```python
from build123d import *

# Parameters (mm, degrees)
F1_DEPTH = 25
F2_SIZE2 = 10
F2_SIZE  = 20
F4_DEPTH = 50
F5_T     = -2.5
F6_R     = 1


with BuildPart() as f1:
    # F0 (on Front) → F1 (new body)
    with BuildSketch(Plane.XZ):
        Polygon((63.5576491768, 36.6950258613), (-63.5576491768, 36.6950258613), (0, -73.3900517225), align=None)
    extrude(amount=-F1_DEPTH)

    # F2
    f2_edges = [f1.edges().sort_by_distance(p)[0] for p in [
        (-31.778825, 25, -18.347513),
        (0, 25, 36.695026),
        (31.778825, 25, -18.347513),
    ]]
    f2_side = f1.faces().sort_by_distance((0, 25, 0))[0]
    chamfer(f2_edges, length=F2_SIZE, length2=F2_SIZE2, reference=f2_side)

    # F3 (on face) → F4 (join, symmetric)
    with BuildSketch(Plane(origin=(0, 25, 0), x_dir=(-1, 0, 0), z_dir=(0, 1, 0))):
        Polygon((-10.3546479691, -5.9782587923), (10.3546479691, -5.9782587923), (0, 11.9565175846), align=None)
    extrude(amount=F4_DEPTH, both=True)

    # F5
    f5_openings = [f1.faces().sort_by_distance(p)[0] for p in [
        (0, -25, 0),
    ]]
    offset(amount=F5_T, openings=f5_openings, kind=Kind.INTERSECTION)

    # F6
    f6_edges = [f1.edges().sort_by_distance(p)[0] for p in [
        (0, -25, -5.978259),
        (0, -25, -3.478259),
        (3.01226, -25, 1.739129),
        (5.177324, -25, 2.989129),
        (-5.177324, -25, 2.989129),
        (-3.01226, -25, 1.739129),
    ]]
    fillet(f6_edges, radius=F6_R)


solid = f1.part
```
Source: CAD feature listing. Evaluate the final solid. Frame: model axes, mm. A direction names the side the tool comes from. Coordinates: 2 decimals unless noted, no trailing zeros. Write each loop counter-clockwise with the first axis right and the second up, starting at its lowest first coordinate (ties: lowest second). Pieces come first, ordered by that corner, then holes. Notation, with made-up numbers: (8, -15.5) - (34, -15.5) arc R9 cw to (34, -0.5) - close; hole circle Ø5 at (-6, 60). An arc over 180 degrees is marked (long way). Answer as a JSON object with one key per item and string values.
Q1. Section query C-C, the plane y = -10.5. Output: boundary loops of the cut face in (x, z).
Ans:
{"outline": "(-10.35, -5.98) - (10.35, -5.98) - (0, 11.96) - close; hole (-6.02, -3.48) - (6.02, -3.48) - (0, 6.96) - close"}
Q2. Section query A-A, the plane x = 19. Output: boundary loops of the cut face in (y, z).
Ans:
{"outline": "(0, -40.48) - (15, -40.48) - (25, -0.48) - (25, 16.7) - (15, 36.7) - (0, 36.7) - close; hole (2.5, -35.48) - (13.45, -35.48) - (22.5, 0.7) - (22.5, 16.1) - (13.45, 34.2) - (2.5, 34.2) - close"}
Q3. Section query D-D, the plane z = -59.5. Output: boundary loops of the cut face in (x, y).
Ans:
{"outline": "(-8.02, 0) - (8.02, 0) - (8.02, 15) - (0, 18.47) - (-8.02, 15) - close; hole (-5.13, 2.5) - (5.13, 2.5) - (5.13, 13.45) - (0, 15.68) - (-5.13, 13.45) - close"}
Q4. Set-up query: faces 4 (the flat face through (2.97, -10.56, 1.81)), 5 (the flat face through (-1, 2.5, -5)), 6 (the flat face through (0.89, 18.819, 29.057)), 7 (the flat face through (0, 50, -5.978)), 8 (the flat face through (0, -12, -5.978)). Return all of +Z, -Z, +X, -X, +Y, -Y with unobstructed straight access to the full face (end or side cutting, diameter ignored); none if empty.
Ans:
{"face 4": "-Y", "face 5": "none", "face 6": "+Z, +X, -X, +Y", "face 7": "-Z, +X, -X, +Y", "face 8": "-Z, +X, -X, -Y"}
Q5. Draft query along Z for faces 1 (the flat face through (23.22, 16.91, -14.36)), 2 (the flat face through (-25.61, 18.82, -13.76)), 3 (the flat face through (-7, 25, 3)). Return one class per face: released by +Z, released by -Z, zero draft, split by the parting line, or undercut.
Ans:
{"face 1": "undercut", "face 2": "released by -Z", "face 3": "zero draft"}
Q6. Material intervals for line 1 (Y direction, x = 8, z = 6); line 2 (Y direction, x = -19.5, z = -13.5); line 3 (Y direction, x = -35, z = -8.5), sorted ascending. Write a range as [from, to].
Ans:
{"line 1": "y = [0, 2.5], [22.5, 25]", "line 2": "y = [0, 2.5], [18.73, 21.53]", "line 3": "y = [0, 16.07]"}
Q7. Section query B-B, the plane z = -16. Output: boundary loops of the cut face in (x, y).
Ans:
{"outline": "(-33.13, 0) - (33.13, 0) - (33.13, 15) - (10.04, 25) - (-10.04, 25) - (-33.13, 15) - close; hole (-30.25, 2.5) - (30.25, 2.5) - (30.25, 13.45) - (9.36, 22.5) - (-9.36, 22.5) - (-30.25, 13.45) - close"}
Q8. First-contact query: pin 1 Ø12 at (x, z) = (18.5, -52.5) entering from +Y; pin 2 Ø16.5 at (x, y) = (-1.5, 50) entering from -Z; pin 3 Ø3.5 at (x, y) = (15, 9.5) entering from -Z. Flat tips, straight axial feed; report the tip coordinate or a pass-through.
Ans:
{"pin 1": "stops at y = 15.21", "pin 2": "stops at z = -5.98", "pin 3": "stops at z = -50.44"}
